The listing builds one solid part. Answer for the finished solid, in the listing's coordinates (mm). Face numbers are marked on the shaded views. Round coordinates to 2 decimals unless told otherwise and drop trailing zeros. Loops run counter-clockwise (first coordinate to the right, second up) from the corner with the lowest first, then second, coordinate; pieces in that order, holes last. Notation, with made-up numbers: (42.5, 83) -> (87.5, 83) arc R16 cw to (87.5, 112) -> close; hole circle Ø11 at (56.5, -18). An arc over 180 degrees is marked (long way). One line per question, with ' | ' between items.
from build123d import *

# Parameters (mm, degrees)
SKETCH_1_W          = 140
SKETCH_1_H          = 80
EXTRUDE_1_DEPTH     = 1
SKETCH_2_W          = 126.458639074
SKETCH_2_H          = 72.505014335
EXTRUDE_2_DEPTH     = 2
SKETCH_3_W          = 121.666196763
SKETCH_3_H          = 67.403382197
CUT_EXTRUDE_1_DEPTH = 0.5


with BuildPart() as part:
    # 草图1 → 凸台-拉伸1 (new body)
    with BuildSketch(Plane(origin=(0, 0, 0), x_dir=(1, 0, 0), z_dir=(0, 1, 0))):
        with Locations((70, -40)):
            Rectangle(SKETCH_1_W, SKETCH_1_H)
    extrude(amount=EXTRUDE_1_DEPTH)

    # 草图2 → 凸台-拉伸2 (add)
    with BuildSketch(Plane(origin=(0, 1, 0), x_dir=(1, 0, 0), z_dir=(0, 1, 0))):
        with Locations((72.164328786, -39.845405087)):
            Rectangle(SKETCH_2_W, SKETCH_2_H)
    extrude(amount=EXTRUDE_2_DEPTH)

    # 草图3 → 切除-拉伸1 (cut)
    with BuildSketch(Plane(origin=(0, 3, 0), x_dir=(1, 0, 0), z_dir=(0, 1, 0))):
        with Locations((72.08703133, -39.458917804)):
            Rectangle(SKETCH_3_W, SKETCH_3_H)
    extrude(amount=-CUT_EXTRUDE_1_DEPTH, mode=Mode.SUBTRACT)


solid = part.part
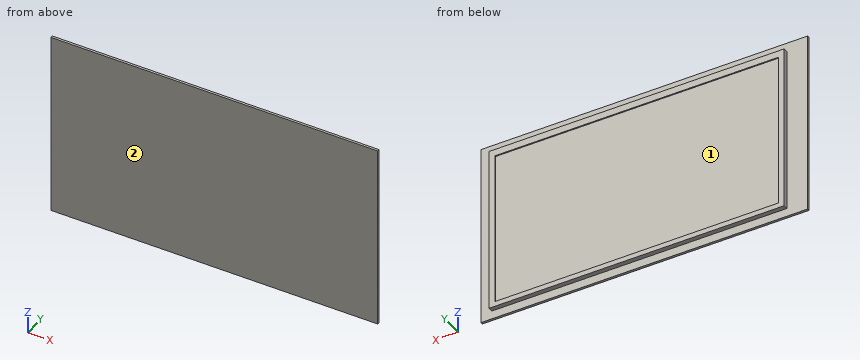
Q1. Given pin 1 Ø1.5 at (x, z) = (16.5, 17) entering from +Y; pin 2 Ø0.6 at (y, z) = (2.5, 49.5) entering from +X; pin 3 Ø0.6 at (x, y) = (79.5, 2) entering from -Z, each flat-ended and moving along its own axis, determine where each tip first touches the part or whether it passes through.
Numbers:
pin 1: y = 2.5 | pin 2: x = 135.39 | pin 3: z = 3.59
Q2. A cutting plane is placed at C-C on y = 1.95. Give the vertices of the cut face in (x, z) (3 decimals).
Numbers:
outline: (8.935, 3.593) -> (135.394, 3.593) -> (135.394, 76.098) -> (8.935, 76.098) -> close
Q3. For a pull along Z with two mould halves and no side action, classify the marked faces 1 and 2 as pulls with the +Z half, pulls with the -Z half, needs draft (parallel to the pull), parting line crosses it, or undercut.
Numbers:
face 1: undercut | face 2: needs draft
Q4. A cutting plane is placed at B-B on z = 61. Give the vertices of the cut face in (x, y) (3 decimals), plus the area to 3 significant figures.
Numbers:
outline: (0, 0) -> (140, 0) -> (140, 1) -> (135.394, 1) -> (135.394, 3) -> (132.92, 3) -> (132.92, 2.5) -> (11.254, 2.5) -> (11.254, 3) -> (8.935, 3) -> (8.935, 1) -> (0, 1) -> close | area: 332 mm^2
Q5. A cutting plane is placed at A-A on x = 111. Give the vertices of the cut face in (y, z), plus the area to 3 significant figures.
Numbers:
outline: (0, 0) -> (1, 0) -> (1, 3.59) -> (3, 3.59) -> (3, 5.76) -> (2.5, 5.76) -> (2.5, 73.16) -> (3, 73.16) -> (3, 76.1) -> (1, 76.1) -> (1, 80) -> (0, 80) -> close | area: 191 mm^2
Q6. Find the intervals of material crossed by line 1 (X direction, y = 2.6, z = 15) (3 decimals); line 2 (Z direction, x = 48, y = 1.9); line 3 (Z direction, x = 24, y = 2.8), in increasing order. Write a range as from..to.
Numbers:
line 1: 8.935..11.254, 132.92..135.394 | line 2: 3.59..76.1 | line 3: 3.59..5.76, 73.16..76.1
